from build123d import *

# Parameters (mm, degrees)
BOSS_EXTRUDE1_DEPTH = 6.35
FILLET2_R           = 10.16


with BuildPart() as part:
    # Sketch1 → Boss-Extrude1 (new body)
    with BuildSketch(Plane(origin=(0, 0, 0), x_dir=(0, 0, -1), z_dir=(1, 0, 0))):
        Polygon((-63.5, -101.6), (-19.05, 50.8), (19.05, 50.8), (63.5, -101.6), align=None)
        with BuildLine():
            ThreePointArc((2.811655808, -13.684132841), (0, 13.97), (-2.811655808, -13.684132841))
            ThreePointArc((-2.811655808, -13.684132841), (0, -21.717), (2.811655808, -13.684132841))
        make_face(mode=Mode.SUBTRACT)
    extrude(amount=BOSS_EXTRUDE1_DEPTH)

    # Fillet2
    fillet2_edges = [part.edges().sort_by_distance(p)[0] for p in [
        (3.175, 50.8, 19.05),
        (3.175, 50.8, -19.05),
    ]]
    fillet(fillet2_edges, radius=FILLET2_R)


solid = part.part
The model under review builds one solid part; all positions refer to its coordinate system, in mm. Round coordinates to 2 decimals unless told otherwise and drop trailing zeros. Loops run counter-clockwise (first coordinate to the right, second up) from the corner with the lowest first, then second, coordinate; pieces in that order, holes last. Notation, with made-up numbers: M 87.25,-32.75 L 93.25,-32.75 A29 cw 93.25,6.25 Z; hole C -17,65 d3. An arc over 180 degrees is marked long. Answer as a JSON object with one key per item and string values.
Item 1: For line 1 along Y through (x, z) = (1.75, 0); line 2 along Y through (x, z) = (5, -11); line 3 along Z through (x, y) = (2.5, 2), list the stretches that pass through material, from the lowest coordinate up.
Check sheet entries:
{"line 1": "-101.6 to -21.72, 13.97 to 50.8", "line 2": "-101.6 to -8.61, 8.61 to 50.8", "line 3": "-33.28 to -13.83, 13.83 to 33.28"}
Item 2: We need section D-D, the plane z = -40. State the section outline as (x, y) points, and give its area (3 significant figures).
Check sheet entries:
{"outline": "M 0,-101.6 L 6.35,-101.6 L 6.35,-21.03 L 0,-21.03 Z", "area": "512 mm2"}
Item 3: The part is to be moulded in two halves that separate along Y. For faces 1 (the face through (3.131, -21.714, 0.156)), 2 (the face through (6.35, -41, -1)), 3 (the face through (3, 50.8, 0)), say which applies: +Y half, -Y half, draft (parallel to the pull), parting line (faces both ways), or undercut.
Check sheet entries:
{"face 1": "undercut", "face 2": "draft", "face 3": "+Y half"}
Item 4: We need section C-C, the plane x = 2.5. State the section outline as (y, z) points.
Check sheet entries:
{"outline": "M -101.6,-63.5 L 43.48,-21.18 A10.16 ccw 50.8,-11.43 L 50.8,11.43 A10.16 ccw 43.48,21.18 L -101.6,63.5 Z; hole M -13.68,-2.81 A13.97 ccw long -13.68,2.81 A4.51 ccw long Z"}
Item 5: We need section A-A, the plane z = 0. State the section outline as (x, y) points, and give its area (3 significant figures).
Check sheet entries:
{"outline": "M 0,-101.6 L 6.35,-101.6 L 6.35,-21.72 L 0,-21.72 Z; M 0,13.97 L 6.35,13.97 L 6.35,50.8 L 0,50.8 Z", "area": "741 mm2"}
Item 6: We need section B-B, the plane y = 0. State the section outline as (x, z) points, and give its area (3 significant figures).
Check sheet entries:
{"outline": "M 0,-33.87 L 6.35,-33.87 L 6.35,-13.97 L 0,-13.97 Z; M 0,13.97 L 6.35,13.97 L 6.35,33.87 L 0,33.87 Z", "area": "253 mm2"}
Item 7: Clearance check with flat-ended pins moving along their axes: P1, Ø8, axis at y = -17.21, z = 0, coming from the +X side; P2, Ø3, axis at x = 1.5, y = 5.5, coming from the +Z side; P3, Ø3, axis at x = 0.5, y = -48, coming from the +Z side. State where each tip first meets the part, or that it passes through.
Check sheet entries:
{"P1": "through", "P2": "z = 32.7", "P3": "z = 48.3"}
